Source: CAD feature listing. Evaluate the final solid. Frame: model axes, mm. A direction names the side the tool comes from. Give positions to 0.01 mm unless a question says otherwise; leave off trailing zeros. Write each loop counter-clockwise with the first axis right and the second up, starting at its lowest first coordinate (ties: lowest second). Pieces come first, ordered by that corner, then holes.
```python
from build123d import *

# Parameters (mm, degrees)
ENL_V_MAT_EXTRU_3_DEPTH = 161.972047263
ESQUISSE8_R             = 9
ENL_V_MAT_EXTRU_4_DEPTH = 161.972047263


with BuildPart() as part:
    # Esquisse6 → Révolution1 (revolve)
    with BuildSketch(Plane.XY):
        with BuildLine():
            Line((0, 21), (0, 33))
            Line((0, 33), (18, 33))
            Line((18, 33), (18, 36))
            Line((18, 36), (20, 36))
            Line((20, 36), (20, 30))
            Line((20, 30), (28, 30))
            Line((28, 30), (28, 36))
            Line((28, 36), (150, 36))
            Line((150, 36), (150, 0))
            Line((150, 0), (80.999999995, 0))
            ThreePointArc((80.999999995, 0), (77.265560701, 9.903895293), (67.921714398, 14.876391154))
            Line((67.921714398, 14.876391154), (36, 19))
            Line((36, 19), (36, 21))
            Line((36, 21), (0, 21))
        make_face()
    revolve(axis=Axis((150, 0, 0), (-1, 0, 0)))

    # Esquisse7 → Enlèv. mat.-Extru.3 (cut, through all)
    with BuildSketch(Plane(origin=(0, 10, 0), x_dir=(1, 0, 0), z_dir=(0, 1, 0))):
        Polygon((105, 36), (84, -36), (150, -36), (150, 36), align=None)
    extrude(amount=-ENL_V_MAT_EXTRU_3_DEPTH, mode=Mode.SUBTRACT)

    # Esquisse8 → Enlèv. mat.-Extru.4 (cut, through all)
    with BuildSketch(Plane(origin=(0, 10, 0), x_dir=(-1, 0, 0), z_dir=(0, 1, 0))):
        with Locations(Location((-132, 0, 0), (0, 0, 180))):
            Circle(ESQUISSE8_R)
        Polygon((-130.288986923, -42.270403954), (-160.663521038, -42.270403954), (-160.663521038, 48.483793559), (-127.12534153, 48.483793559), (-150, 0), align=None)
    extrude(amount=ENL_V_MAT_EXTRU_4_DEPTH, mode=Mode.SUBTRACT)


solid = part.part
```
1. Access query for faces 4 (the flat face through (20, -14, -27)), 5 (the cylindrical face through (9.1, 30.5, 12.6)), 6 (the flat face through (117, 10, 0)). Directions: +Z, -Z, +X, -X, +Y, -Y. A direction counts if a zero-diameter tool reaches every point of the face in a straight line with its end or side. Return the directions, or none.
2. Line query: L1, parallel to Y at x = 11, z = 0; L2, parallel to Y at x = 56.5, z = 0. Output: solid intervals per line, ascending.
3. Cut plane A-A, the plane x = 132. Return the cut outline in (y, z).
4. Cut plane B-B, the plane y = 27. Return the cut outline in (x, z).
5. Contact query for flat-ended pins moving along their axis: P1, Ø8, axis at x = 83, z = -17.5, coming from the +Y side; P2, Ø5, axis at x = 108, y = 15, coming from the +Z side; P3, Ø4, axis at x = 15.5, z = 8.5, coming from the +Y side; P4, Ø16, axis at x = 132, z = 0, coming from the +Y side. Output: stop coordinate, or through.
6. Mould query, pull axis Y, two halves, no side actions, for faces 1 (the cylindrical face through (17.75, 20.03, -6.31)), 2 (the cylindrical face through (19.014, -4.686, -35.694)), 3 (the cylindrical face through (140.314, 22.818, 3.447)). Classes: +Y half, -Y half, draft (parallel to the pull), parting line (faces both ways), or undercut.
7. Cut plane C-C, the plane x = 22. Return the cut outline in (y, z).
8. Cut plane D-D, the plane z = -24.5. Return the cut outline in (x, y), then the cut area to 3 significant figures.
Response values:
1. face 4: none
1. face 5: -X
1. face 6: +Z, +X, -Y
2. L1: y = -33 to -21, 21 to 33
2. L2: y = -36 to -16.35, 16.35 to 36
3. outline: (10, -34.58) arc R36 ccw to (34.86, -9) - (10, -9) - close; (10, 9) - (34.86, 9) arc R36 ccw to (10, 34.58) - close
4. outline: (0, -18.97) - (18, -18.97) - (18, -23.81) - (20, -23.81) - (20, -13.08) - (28, -13.08) - (28, -23.81) - (138.9, -23.81) - (150, 0) - (138.77, 23.81) - (28, 23.81) - (28, 13.08) - (20, 13.08) - (20, 23.81) - (18, 23.81) - (18, 18.97) - (0, 18.97) - close; hole circle Ø18 at (132, 0)
5. P1: stops at y = 33.37
5. P2: stops at z = 33.76
5. P3: stops at y = 32.35
5. P4: passes through
6. face 1: undercut
6. face 2: parting line
6. face 3: draft
7. outline: circle Ø60 at (0, 0); hole circle Ø42 at (0, 0)
8. outline: (0, -22.11) - (18, -22.11) - (18, -26.38) - (20, -26.38) - (20, -17.31) - (28, -17.31) - (28, -26.38) - (101.65, -26.38) - (101.65, 10) - (138.58, 10) - (138.58, 26.38) - (28, 26.38) - (28, 17.31) - (20, 17.31) - (20, 26.38) - (18, 26.38) - (18, 22.11) - (0, 22.11) - close
8. area: 5,670 mm2
